Verification items for the finished model (mm, model axes). Face numbers are marked on the shaded views. A direction names the side the tool comes from. Coordinates: 2 decimals unless noted, no trailing zeros. Loops run counter-clockwise (first coordinate to the right, second up) from the corner with the lowest first, then second, coordinate; pieces in that order, holes last.
Q1. Access from +Z, -Z, +X, -X, +Y, -Y to the whole of each face (thin tool, end or side, straight path). Record for the marked faces 4, 5 and 6.
Q2. Mould release check, pull along Z, two halves, no side actions. Record for the marked faces 1, 2 and 3: +Z half, -Z half, draft (parallel to the pull), parting line (faces both ways), or undercut.
Q3. Go/stop test with flat-tipped pins: P1, Ø5, axis at y = -15.5, z = 21, coming from the -X side; P2, Ø1.5, axis at y = 28.5, z = -0.5, coming from the +X side; P3, Ø8, axis at y = 21.5, z = 15.5, coming from the -X side; P4, Ø1.5, axis at y = -16.5, z = 33.5, coming from the +X side. Record where each tip stops, or that it passes through.
Q4. Sectioned sample at A-A (x = 0). Enter the section's corners in (y, z), then the cut area to 3 significant figures.
Q5. Material ranges on probe 1 along Y at (x, z) = (0, -13.5); probe 2 along Z at (x, y) = (4.25, 0); probe 3 along X at (y, z) = (4, 32), recorded low to high.
Q6. Sectioned sample at B-B (y = 2). Enter the section's corners in (x, z).
Q7. Sectioned sample at C-C (z = 55). Enter the section's corners in (x, y), then the cut area to 3 significant figures.
Q8. Sectioned sample at D-D (y = -13). Enter the section's corners in (x, z).
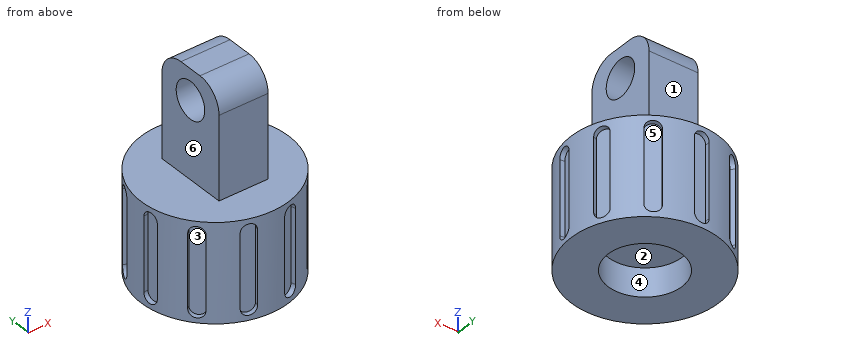
```python
from build123d import *

# Parameters (mm, degrees)
SKETCH1_R               = 30
BOSS_EXTRUDE1_DEPTH     = 20
SKETCH2_W               = 43.772926879
SKETCH2_H               = 30
BOSS_EXTRUDE2_DEPTH     = 10
FILLET1_R               = 10
CUT_EXTRUDE1_DEPTH      = 82.036943444
CUT_EXTRUDE1_DEPTH_BACK = 82.036943444
SKETCH3_R               = 7.5
CUT_EXTRUDE2_START      = 28
CUT_EXTRUDE2_DEPTH      = 20
CIRPATTERN1_COUNT       = 11
SKETCH5_R               = 15
CUT_EXTRUDE3_DEPTH      = 11.5


with BuildPart() as part:
    # Sketch1 → Boss-Extrude1 (new, symmetric)
    with BuildSketch(Plane.XY):
        Circle(SKETCH1_R)
    extrude(amount=BOSS_EXTRUDE1_DEPTH, both=True)

    # Sketch2 → Boss-Extrude2 (add, symmetric)
    with BuildSketch(Plane(origin=(0, 0, 0), x_dir=(0, 0, -1), z_dir=(1, 0, 0))):
        with Locations((-41.88646344, 0)):
            Rectangle(SKETCH2_W, SKETCH2_H)
    extrude(amount=BOSS_EXTRUDE2_DEPTH, both=True)

    # Fillet1
    fillet1_edges = [part.edges().sort_by_distance(p)[0] for p in [
        (0, 15, 63.772926879),
        (0, -15, 63.772926879),
    ]]
    fillet(fillet1_edges, radius=FILLET1_R)

    # Sketch3 → Cut-Extrude1 (cut, two sides: drawn at the far end of the back side and taken through both)
    with BuildSketch(Plane(origin=(10, 0, 0), x_dir=(0, 0, -1), z_dir=(1, 0, 0)).offset(-CUT_EXTRUDE1_DEPTH_BACK)):
        with Locations((-51.35721853, 0)):
            Circle(SKETCH3_R)
    extrude(amount=CUT_EXTRUDE1_DEPTH + CUT_EXTRUDE1_DEPTH_BACK, mode=Mode.SUBTRACT)

    # Sketch4 → Cut-Extrude2 (cut)
    with BuildSketch(Plane(origin=(0, 0, 0), x_dir=(1, 0, 0), z_dir=(0, 1, 0)).offset(CUT_EXTRUDE2_START)):
        with BuildLine():
            Line((3, 15), (3, -15))
            ThreePointArc((3, -15), (0, -18), (-3, -15))
            Line((-3, -15), (-3, 15))
            ThreePointArc((-3, 15), (0, 18), (3, 15))
        make_face()
    cut_extrude2 = extrude(amount=CUT_EXTRUDE2_DEPTH, mode=Mode.SUBTRACT)

    # CirPattern1: Cut-Extrude2 ×11 about axis
    cirpattern1_axis = Axis((0, 0, 0), (0, 0, 1))
    for i in range(1, CIRPATTERN1_COUNT):
        add(cut_extrude2.rotate(cirpattern1_axis, i * 360 / CIRPATTERN1_COUNT), mode=Mode.SUBTRACT)

    # Sketch5 → Cut-Extrude3 (cut)
    with BuildSketch(Plane(origin=(0, 0, -20), x_dir=(-1, 0, 0), z_dir=(0, 0, -1))):
        Circle(SKETCH5_R)
    extrude(amount=-CUT_EXTRUDE3_DEPTH, mode=Mode.SUBTRACT)


solid = part.part
```
Geometry check:
1. face 4: -Z
1. face 5: none
1. face 6: +Z, -X, +Y, -Y
2. face 1: draft
2. face 2: -Z half
2. face 3: undercut
3. P1: stops at x = -26.94
3. P2: stops at x = 11.4
3. P3: stops at x = -24.37
3. P4: passes through
4. outline: (-30, -20) - (-15, -20) - (-15, -8.5) - (15, -8.5) - (15, -20) - (30, -20) - (30, -18) - (28, -18) - (28, 18) - (30, 18) - (30, 20) - (15, 20) - (15, 53.77) arc R10 ccw to (5, 63.77) - (-5, 63.77) arc R10 ccw to (-15, 53.77) - (-15, 20) - (-30, 20) - close; hole circle Ø15 at (0, 51.36)
4. area: 3,080 mm2
5. probe 1: y = -30 to -15, 15 to 28
5. probe 2: z = -8.5 to 43.86, 58.86 to 63.77
5. probe 3: x = -10 to 10
6. outline: (-29.93, -20) - (-14.87, -20) - (-14.87, -8.5) - (14.87, -8.5) - (14.87, -20) - (29.93, -20) - (29.93, 20) - (10, 20) - (10, 44.13) - (-10, 44.13) - (-10, 20) - (-29.93, 20) - close; (-10, 58.59) - (10, 58.59) - (10, 63.77) - (-10, 63.77) - close
7. outline: (-10, -14.92) - (10, -14.92) - (10, -6.56) - (-10, -6.56) - close; (-10, 6.56) - (10, 6.56) - (10, 14.92) - (-10, 14.92) - close
7. area: 335 mm2
8. outline: (-27.04, -20) - (-7.48, -20) - (-7.48, -8.5) - (7.48, -8.5) - (7.48, -20) - (27.04, -20) - (27.04, 20) - (10, 20) - (10, 59.77) - (-10, 59.77) - (-10, 20) - (-27.04, 20) - close
